For this review, take the finished solid that the model builds, in its own axes (mm). A direction names the side the tool comes from. Round coordinates to 2 decimals unless told otherwise and drop trailing zeros. Loops run counter-clockwise (first coordinate to the right, second up) from the corner with the lowest first, then second, coordinate; pieces in that order, holes last. Notation, with made-up numbers: (36, -7.5) -> (42, -7.5) arc R29 cw to (42, 26.5) -> close; hole circle Ø9 at (3, -13.75). An arc over 180 degrees is marked (long way). Write each question's results on one line, items separated by ' | '.
```python
from build123d import *

# Parameters (mm, degrees)
BOSS_EXTRUDE1_DEPTH = 12.5
CUT_EXTRUDE1_DEPTH  = 46.356917885


with BuildPart() as part:
    # Sketch1 → Boss-Extrude1 (new, symmetric)
    with BuildSketch(Plane(origin=(0, 0, 0), x_dir=(1, 0, 0), z_dir=(0, 1, 0))):
        with BuildLine():
            Line((0, 13), (35, 13))
            Line((35, 13), (35, 9))
            Line((35, 9), (0, 9))
            ThreePointArc((0, 9), (-6.363961031, 6.363961031), (-9, 0))
            ThreePointArc((-9, 0), (-6.363961031, -6.363961031), (0, -9))
            Line((0, -9), (35, -9))
            Line((35, -9), (35, -13))
            Line((35, -13), (0, -13))
            ThreePointArc((0, -13), (-9.192388155, -9.192388155), (-13, 0))
            ThreePointArc((-13, 0), (-9.192388155, 9.192388155), (0, 13))
        make_face()
    extrude(amount=BOSS_EXTRUDE1_DEPTH, both=True)

    # Sketch2 → Cut-Extrude1 (cut, through all)
    with BuildSketch(Plane.XY.offset(13)):
        with BuildLine():
            ThreePointArc((27.5, 0), (22.5, 5), (17.5, 0))
            Line((17.5, 0), (27.5, 0))
        make_face()
        with BuildLine():
            Line((27.5, 0), (17.5, 0))
            ThreePointArc((17.5, 0), (22.5, -5), (27.5, 0))
        make_face()
        with BuildLine():
            ThreePointArc((22.5, 12.5), (31.338834755, 8.838834775), (35, 2.9e-08))
            Line((35, 2.9e-08), (35, 12.5))
            Line((35, 12.5), (22.5, 12.5))
        make_face()
        with BuildLine():
            Line((35, -12.5), (35, 2.9e-08))
            ThreePointArc((35, 2.9e-08), (31.338834775, -8.838834755), (22.5, -12.5))
            Line((22.5, -12.5), (35, -12.5))
        make_face()
    extrude(amount=-CUT_EXTRUDE1_DEPTH, mode=Mode.SUBTRACT)


solid = part.part
```
1. Tool access review of faces 4 (the face through (0, -12.5, 10)), 5 (the face through (17, 0, 9)): name each direction out of +Z, -Z, +X, -X, +Y, -Y from which nothing blocks a thin tool from reaching the whole face with its end or side.
Values found:
face 4: +Z, -Z, +X, -X, -Y | face 5: +X, +Y, -Y
2. Consider section D-D (x = 23). State the section outline as (y, z) points, plus the area to 3 significant figures.
Values found:
outline: (-12.49, -13) -> (-4.97, -13) -> (-4.97, -9) -> (-12.49, -9) -> close; (-12.49, 9) -> (-4.97, 9) -> (-4.97, 13) -> (-12.49, 13) -> close; (4.97, -13) -> (12.49, -13) -> (12.49, -9) -> (4.97, -9) -> close; (4.97, 9) -> (12.49, 9) -> (12.49, 13) -> (4.97, 13) -> close | area: 120 mm2
3. Consider section C-C (y = 8). State the section outline as (x, z) points, plus the area to 3 significant figures.
Values found:
outline: (0, -13) -> (32.1, -13) -> (32.1, -9) -> (0, -9) arc R9 cw to (0, 9) -> (32.1, 9) -> (32.1, 13) -> (0, 13) arc R13 ccw to start | area: 395 mm2
4. Consider section B-B (y = -2.5). State the section outline as (x, z) points.
Values found:
outline: (0, -13) -> (18.17, -13) -> (18.17, -9) -> (0, -9) arc R9 cw to (0, 9) -> (18.17, 9) -> (18.17, 13) -> (0, 13) arc R13 ccw to start; (26.83, -13) -> (34.75, -13) -> (34.75, -9) -> (26.83, -9) -> close; (26.83, 9) -> (34.75, 9) -> (34.75, 13) -> (26.83, 13) -> close
5. To check wall thickness, follow probe 1 along Y at (x, z) = (22.5, 11.95); probe 2 along Z at (x, y) = (21, 5.5); probe 3 along Z at (x, y) = (-5.5, -2.75). State the ranges of each line that lie inside material, in increasing order.
Values found:
probe 1: y = -12.5 to -5, 5 to 12.5 | probe 2: z = -13 to -9, 9 to 13 | probe 3: z = -11.78 to -7.12, 7.12 to 11.78
6. Consider section A-A (x = 7). State the section outline as (y, z) points.
Values found:
outline: (-12.5, -13) -> (12.5, -13) -> (12.5, -9) -> (-12.5, -9) -> close; (-12.5, 9) -> (12.5, 9) -> (12.5, 13) -> (-12.5, 13) -> close
7. For pin 1 (1.5 mm diameter, centred on y = 4, z = 4, fed in from +X); pin 2 (6 mm diameter, centred on y = -9, z = -1.5, fed in from -X), all flat-tipped, find the tip position at first contact; note any pin that passes through.
Values found:
pin 1: stops at x = -7.64 | pin 2: stops at x = -13
8. Draft analysis for pull direction X (two halves, no side actions). For faces 1 (the face through (-9, 0, 0)), 2 (the face through (0, 12.5, 10)), 3 (the face through (27.495, -0.22, -10.972)), state which applies: released by +X, released by -X, zero draft, split by the parting line, or undercut.
Values found:
face 1: released by +X | face 2: zero draft | face 3: undercut
